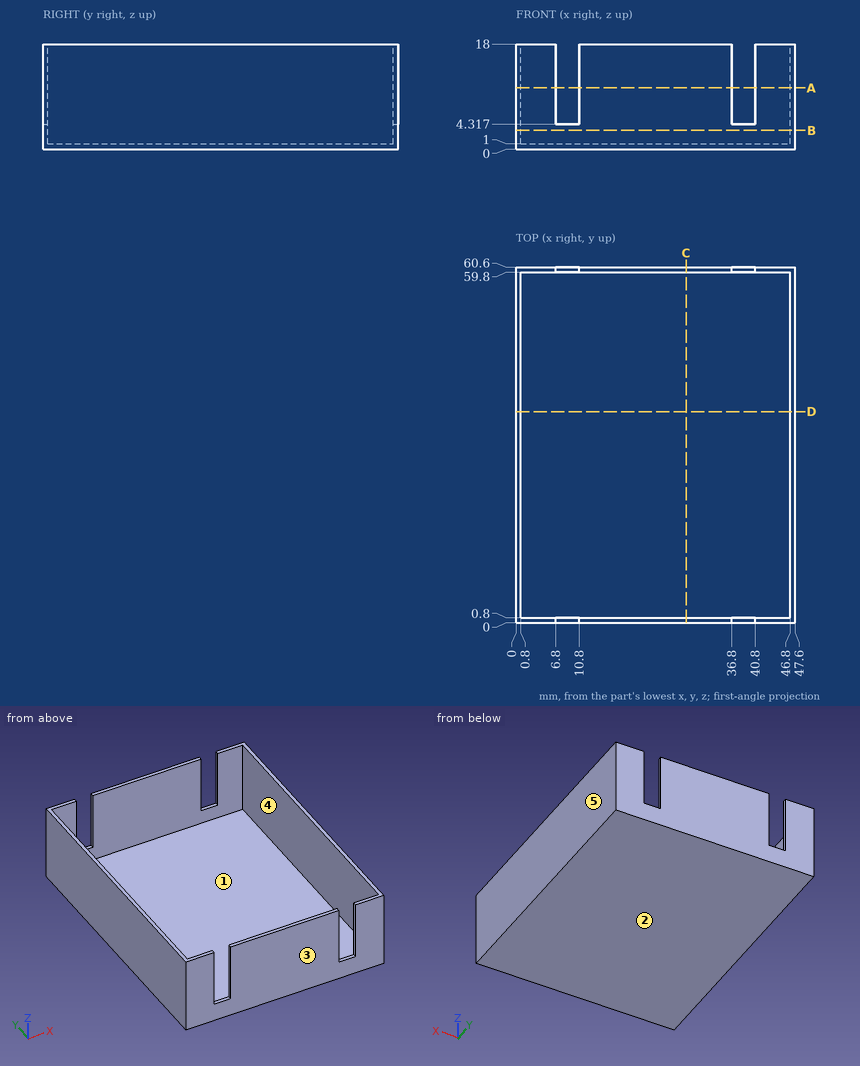
Design review of the part shown in the three views and the two pictorial views. Dimensions are in mm from the part's minimum x, y and z. A direction names the side the tool comes from. Round coordinates to 2 decimals unless told otherwise and drop trailing zeros. Order: outer loops, then holes, each group sorted by start corner. A loop starts at its lowest first (then second) coordinate and runs counter-clockwise, first axis right, second up.
Item 1: Machinability: for the marked faces 4 and 5, which of the approach directions +Z, -Z, +X, -X, +Y, -Y give a long, thin tool a straight path to every point of the face, cutting with its end or side? Answer none if there is none.
Working result:
face 4: +Z
face 5: +Z, -Z, +X, +Y, -Y
Item 2: Add section C-C, the plane x = 29. State the section outline as (y, z) points, and give its area (3 significant figures).
Working result:
outline: (0, 0) - (60.6, 0) - (60.6, 18) - (59.8, 18) - (59.8, 1) - (0.8, 1) - (0.8, 18) - (0, 18) - close
area: 87.8 mm2
Item 3: Draft analysis for pull direction Y (two halves, no side actions). For the marked faces 1, 2 and 3, state which applies: released by +Y, released by -Y, zero draft, split by the parting line, or undercut.
Working result:
face 1: undercut
face 2: zero draft
face 3: released by -Y
Item 4: Add section B-B, the plane z = 3.25. State the section outline as (x, y) points, and give its area (3 significant figures).
Working result:
outline: (0, 0) - (47.6, 0) - (47.6, 60.6) - (0, 60.6) - close; hole (0.8, 0.8) - (46.8, 0.8) - (46.8, 59.8) - (0.8, 59.8) - close
area: 171 mm2
Item 5: Add section D-D, the plane y = 36. State the section outline as (x, z) points.
Working result:
outline: (0, 0) - (47.6, 0) - (47.6, 18) - (46.8, 18) - (46.8, 1) - (0.8, 1) - (0.8, 18) - (0, 18) - close
Item 6: To check wall thickness, follow probe 1 along Y at (x, z) = (29, 12); probe 2 along X at (y, z) = (22.5, 8.5); probe 3 along Z at (x, y) = (24.5, 43). State the ranges of each line that lie inside material, in increasing order.
Working result:
probe 1: y = 0 to 0.8, 59.8 to 60.6
probe 2: x = 0 to 0.8, 46.8 to 47.6
probe 3: z = 0 to 1
Item 7: Add section A-A, the plane z = 10.5. State the section outline as (x, y) points, and give its area (3 significant figures).
Working result:
outline: (0, 0) - (6.8, 0) - (6.8, 0.8) - (0.8, 0.8) - (0.8, 59.8) - (6.8, 59.8) - (6.8, 60.6) - (0, 60.6) - close; (10.8, 0) - (36.8, 0) - (36.8, 0.8) - (10.8, 0.8) - close; (10.8, 59.8) - (36.8, 59.8) - (36.8, 60.6) - (10.8, 60.6) - close; (40.8, 0) - (47.6, 0) - (47.6, 60.6) - (40.8, 60.6) - (40.8, 59.8) - (46.8, 59.8) - (46.8, 0.8) - (40.8, 0.8) - close
area: 158 mm2
Item 8: For pin 1 (0.6 mm diameter, centred on x = 38, y = 60.5, fed in from +Z); pin 2 (14 mm diameter, centred on x = 25, y = 42.5, fed in from +Z), all flat-tipped, find the tip position at first contact; note any pin that passes through.
Working result:
pin 1: stops at z = 4.32
pin 2: stops at z = 1
